Build history of the part. All positions in model axes, mm. A direction names the side the tool comes from. Give positions to 0.01 mm unless a question says otherwise; leave off trailing zeros. Order: outer loops, then holes, each group sorted by start corner. A loop starts at its lowest first (then second) coordinate and runs counter-clockwise, first axis right, second up. Notation, with made-up numbers: (11.25, -2.5) -> (64.25, -2.5) arc R12 ccw to (64.25, 20.5) -> close; hole circle Ø5 at (-13, -4.5). An arc over 180 degrees is marked (long way). One line per item, written item: value. Start each with the question number.
(1) Saw through at A-A on y = 2.5. Give the cut face in (x, z), plus the area to 3 significant figures.
(2) Saw through at D-D on y = -4. Give the cut face in (x, z), plus the area to 3 significant figures.
(3) Pin check, flat tips, straight feed: pin 1 (3 mm diameter, centred on x = 1.5, y = -3, fed in from +Z); pin 2 (1.2 mm diameter, centred on y = 1, z = 2, fed in from -X). Stop position of each tip, or through.
(4) Which spindle directions (+Z, -Z, +X, -X, +Y, -Y) get a long thin tool onto all of the face, cutting with end or side? Do faces 1 (the cylindrical face through (0.63, -0.45, 5)), 2 (the flat face through (45, 0, 3)), 3 (the flat face through (-45, 0, 3)). Say none if no direction does.
(5) Probe line 1 (X direction, y = 0.25, z = 2.6); line 2 (Z direction, x = -29.5, y = -5.5); line 3 (Z direction, x = -41, y = 1.75). List the from-to ranges inside material, lowest first.
(6) Saw through at C-C on z = 3.65. Give the cut face in (x, y), plus the area to 3 significant figures.
(7) Saw through at B-B on x = -3.5. Give the cut face in (y, z).
```python
from build123d import *

# Parameters (mm, degrees)
F0_W     = 100
F0_H     = 15
F1_DEPTH = 1
F2_W     = 90
F2_H     = 5
F3_ANGLE = 180


with BuildPart() as f1:
    # F0 (on Top) → F1 (new body)
    with BuildSketch(Plane.XY):
        Rectangle(F0_W, F0_H)
    extrude(amount=F1_DEPTH)

    # F2 (on Top) → F3 (revolve)
    with BuildSketch(Plane.XY):
        with Locations((0, -2.855439)):
            Rectangle(F2_W, F2_H)
    revolve(axis=Axis((0, -0.355439, 0), (-1, 0, 0)), revolution_arc=F3_ANGLE)


solid = f1.part
```
Results below:
1. outline: (-50, 0) -> (50, 0) -> (50, 1) -> (45, 1) -> (45, 4.1) -> (-45, 4.1) -> (-45, 1) -> (-50, 1) -> close
1. area: 379 mm²
2. outline: (-50, 0) -> (50, 0) -> (50, 1) -> (45, 1) -> (45, 3.42) -> (-45, 3.42) -> (-45, 1) -> (-50, 1) -> close
2. area: 318 mm²
3. pin 1: stops at z = 4.87
3. pin 2: stops at x = -45
4. face 1: +Z, +X, -X
4. face 2: +Z, +X, +Y, -Y
4. face 3: +Z, -X, +Y, -Y
5. line 1: x = -45 to 45
5. line 2: z = 0 to 1
5. line 3: z = 0 to 4.54
6. outline: (-45, -3.77) -> (45, -3.77) -> (45, 3.06) -> (-45, 3.06) -> close
6. area: 615 mm²
7. outline: (-7.5, 0) -> (7.5, 0) -> (7.5, 1) -> (4.54, 1) arc R5 ccw to (-5.25, 1) -> (-7.5, 1) -> close
